Verification items for the finished model (mm, model axes). A direction names the side the tool comes from. Give positions to 0.01 mm unless a question says otherwise; leave off trailing zeros. Order: outer loops, then holes, each group sorted by start corner. A loop starts at its lowest first (then second) coordinate and runs counter-clockwise, first axis right, second up. Notation, with made-up numbers: (33.5, -18.5) - (84.5, -18.5) arc R31 cw to (84.5, 8.5) - close; hole circle Ø10 at (60, -22). An arc over 180 degrees is marked (long way). Answer as a JSON object with one key per item and string values.
Autodesk Inventor part; units mm, degrees
ref_plane "YZ Plane" through (0, 0, 0) normal (1, 0, 0) x (0, 1, 0)
ref_plane "XZ Plane" through (0, 0, 0) normal (0, 1, 0) x (-1, 0, 0)
ref_plane "XY Plane" through (0, 0, 0) normal (0, 0, 1) x (1, 0, 0)
sketch "스케치1" plane through (0, 0, 0) normal (0, 1, 0) x (-1, 0, 0)
  circle A0 centre (0, 0) radius 4.35
  circle A1 centre (0, 0) radius 2.75
  dimension "d0" = 8.7
  dimension "d1" = 5.5
extrude "돌출1" add sketch "스케치1" against normal blind 3
sketch "스케치3" plane through (0, 0, 0) normal (0, 1, 0) x (1, 0, 0)
  circle A0 centre (0, 0) radius 10.5
  circle A1 centre (0, 0) radius 1.5
  dimension "d4" = 21
  dimension "d5" = 3
extrude "돌출2" add sketch "스케치3" along normal blind 2.2
sketch "스케치4" plane through (0, 2.2, 0) normal (0, 1, 0) x (1, 0, 0)
  circle A0 centre (0, 0) radius 2.85
  circle A1 centre (0, 0) radius 3.05
  circle A2 centre (0, 0) radius 4.25
  dimension "d8" = 5.7
  dimension "d9" = 6.1
  dimension "d10" = 8.5
extrude "돌출3" cut sketch "스케치4" against normal blind 1
sketch "스케치5" plane through (0, 2.2, 0) normal (0, 1, 0) x (1, 0, 0)
  circle A0 centre (-7, 0) radius 1
  circle A1 centre (-7, -3.5) radius 1
  line L0 (0, 0) -> (-0.944, 0)
  circle A2 centre (-7, 3.5) radius 1
  dimension "d13" = 2
  dimension "d14" = 7
  dimension "d15" = 2
  dimension "d16" = 3.5
extrude "돌출4" cut sketch "스케치5" against normal blind 7.25
pattern_circular "원형 패턴1" count 4 over 360 about axis through (0, 2.2, 0) along (0, -1, 0) of "돌출4"
properties part number "MG서보모터 원형부품"
(1) Material ranges on line 1 along X through (y, z) = (0.85, 6.75); line 2 along X through (y, z) = (0.4, -3.25); line 3 along X through (y, z) = (0.6, -7.5), recorded low to high. Write a range as [from, to].
Computed values:
{"line 1": "x = [-8.04, -4.47], [-2.53, -0.97], [0.97, 2.53], [4.47, 8.04]", "line 2": "x = [-9.98, -7.97], [-6.03, 6.03], [7.97, 9.98]", "line 3": "x = [-7.35, -4.37], [-2.63, -0.87], [0.87, 2.63], [4.37, 7.35]"}
(2) Gauge pin test, flat ends, axial feed: pin 1 Ø1.8 at (x, z) = (7, 0) entering from +Y; pin 2 Ø2.5 at (x, z) = (-3.5, 7) entering from -Y; pin 3 Ø1.5 at (y, z) = (-2, -1.5) entering from -X. Record the tip position at first contact, or that the pin passes through.
Computed values:
{"pin 1": "passes through", "pin 2": "stops at y = 0", "pin 3": "stops at x = -4.28"}
(3) Section check A-A (y = 0.3). Count the separate pieces of the cut face and the enclosed holes in it, then the cut area to 3 significant figures.
Computed values:
{"separate pieces": "1", "enclosed holes": "13", "area": "302 mm²"}
(4) Section check D-D (z = -3.5). Record the cut outline in (x, y).
Computed values:
{"outline": "(-9.9, 0) - (-8, 0) - (-8, 2.2) - (-9.9, 2.2) - close; (-6, 0) - (-2.58, 0) - (-2.58, -3) - (2.58, -3) - (2.58, 0) - (6, 0) - (6, 2.2) - (2.41, 2.2) - (2.41, 1.2) - (-2.41, 1.2) - (-2.41, 2.2) - (-6, 2.2) - close; (8, 0) - (9.9, 0) - (9.9, 2.2) - (8, 2.2) - close"}
(5) Section check B-B (x = 4). Record the cut outline in (y, z).
Computed values:
{"outline": "(-3, -1.71) - (0, -1.71) - (0, -6.13) - (2.2, -6.13) - (2.2, -1.44) - (1.2, -1.44) - (1.2, 1.44) - (2.2, 1.44) - (2.2, 6.13) - (0, 6.13) - (0, 1.71) - (-3, 1.71) - close; (0, -9.71) - (2.2, -9.71) - (2.2, -7.87) - (0, -7.87) - close; (0, 7.87) - (2.2, 7.87) - (2.2, 9.71) - (0, 9.71) - close"}
(6) Section check C-C (z = -7.75). Record the cut outline in (x, y), then the cut area to 3 significant figures.
Computed values:
{"outline": "(-7.08, 0) - (-4.16, 0) - (-4.16, 2.2) - (-7.08, 2.2) - close; (-2.84, 0) - (-0.66, 0) - (-0.66, 2.2) - (-2.84, 2.2) - close; (0.66, 0) - (2.84, 0) - (2.84, 2.2) - (0.66, 2.2) - close; (4.16, 0) - (7.08, 0) - (7.08, 2.2) - (4.16, 2.2) - close", "area": "22.4 mm²"}
(7) Release check for a two-part mould opening along Z. For faces 1 (the flat face through (2, 1.2, 3)), 2 (the cylindrical face through (10, 1.1, 3.2)), 3 (the cylindrical face through (-1.5, 0.59, 0.07)), 4 (the flat face through (5, 2.2, 0)) record: pulls with the +Z half, pulls with the -Z half, needs draft (parallel to the pull), parting line crosses it, or undercut.
Computed values:
{"face 1": "undercut", "face 2": "parting line crosses it", "face 3": "undercut", "face 4": "needs draft"}
(8) Access from +Z, -Z, +X, -X, +Y, -Y to the whole of each face (thin tool, end or side, straight path). Record for faces 5 (the cylindrical face through (-3.047, 1.707, -0.134)), 6 (the cylindrical face through (0.596, -1.479, -2.685)), 7 (the cylindrical face through (0.6, 1.1, 7.8)).
Computed values:
{"face 5": "+Y", "face 6": "-Y", "face 7": "+Y, -Y"}
